from build123d import *

# Parameters (mm, degrees)
SKETCH1_W           = 97.5
SKETCH1_H           = 45.5
SKETCH1_W_2         = 93.5
SKETCH1_H_2         = 41.5
BOSS_EXTRUDE1_DEPTH = 4
SKETCH2_W           = 102.5
SKETCH2_H           = 50.5
BOSS_EXTRUDE2_DEPTH = 4
CUT_EXTRUDE1_DEPTH  = 58.689903796


with BuildPart() as part:
    # Sketch1 → Boss-Extrude1 (new body)
    with BuildSketch(Plane(origin=(0, 0, 0), x_dir=(1, 0, 0), z_dir=(0, 1, 0))):
        Rectangle(SKETCH1_W, SKETCH1_H)
        Rectangle(SKETCH1_W_2, SKETCH1_H_2, mode=Mode.SUBTRACT)
    extrude(amount=BOSS_EXTRUDE1_DEPTH)

    # Sketch2 → Boss-Extrude2 (add)
    with BuildSketch(Plane(origin=(0, 0, 0), x_dir=(-1, 0, 0), z_dir=(0, -1, 0))):
        Rectangle(SKETCH2_W, SKETCH2_H)
    extrude(amount=BOSS_EXTRUDE2_DEPTH)

    # Sketch3 → Cut-Extrude1 (cut, through all)
    with BuildSketch(Plane.XZ.offset(4)):
        with BuildLine():
            Line((21.754778505, -2.585841929), (14.396321324, 4.772615252))
            ThreePointArc((14.396321324, 4.772615252), (3.257355265, -2.585841929), (14.396321324, -9.94429911))
            Line((14.396321324, -9.94429911), (21.754778505, -2.585841929))
        make_face()
        with BuildLine():
            ThreePointArc((27.699814048, 16.344452811), (17.739587878, 15.654593104), (16.208809841, 5.78855386))
            Line((16.208809841, 5.78855386), (23.168992067, -1.171628366))
            Line((23.168992067, -1.171628366), (30.046481727, 5.705861294))
            ThreePointArc((30.046481727, 5.705861294), (31.14634131, 10.054344559), (29.732993239, 14.31127362))
            Line((29.732993239, 14.31127362), (27.699814048, 16.344452811))
        make_face()
        with BuildLine():
            ThreePointArc((15.482875978, -11.68617158), (23.435669898, -22.607420615), (29.929242502, -10.760305926))
            Line((29.929242502, -10.760305926), (23.168992067, -4.000055491))
            Line((23.168992067, -4.000055491), (15.482875978, -11.68617158))
        make_face()
        with BuildLine():
            ThreePointArc((40.538950668, 3.505316191), (36.33465085, 5.37848968), (31.79403897, 4.624991411))
            Line((31.79403897, 4.624991411), (24.58320563, -2.585841929))
            Line((24.58320563, -2.585841929), (31.677379035, -9.680015334))
            ThreePointArc((31.677379035, -9.680015334), (41.608009289, -7.500810005), (41.380693911, 2.663572949))
            Line((41.380693911, 2.663572949), (40.538950668, 3.505316191))
        make_face()
        with BuildLine():
            Line((-31.75, 0.342207976), (-38.75, 0.422889955))
            ThreePointArc((-38.75, 0.422889955), (-46.75, -7.577110045), (-38.75, -15.577110045))
            Line((-38.75, -15.577110045), (-8.75, -15.75))
            ThreePointArc((-8.75, -15.75), (-0.75, -7.75), (-8.75, 0.25))
            Line((-8.75, 0.25), (-15.75, 0.25))
            Line((-15.75, 0.25), (-15.75, 7.75))
            ThreePointArc((-15.75, 7.75), (-23.75, 15.75), (-31.75, 7.75))
            Line((-31.75, 7.75), (-31.75, 0.342207976))
        make_face()
    extrude(amount=-CUT_EXTRUDE1_DEPTH, mode=Mode.SUBTRACT)


solid = part.part
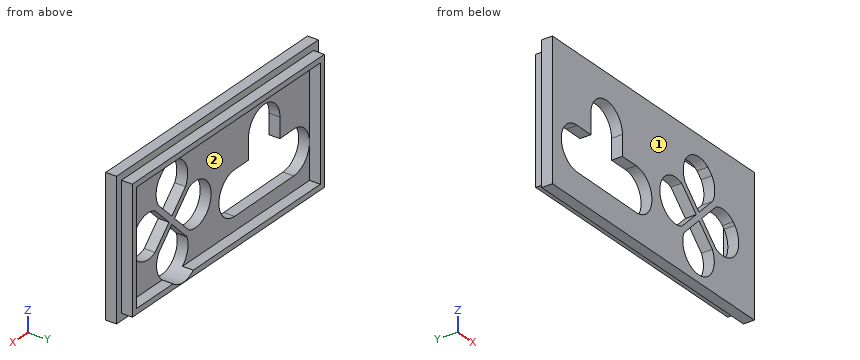
Build history of the part. All positions in model axes, mm. Face numbers are marked on the shaded views. Give positions to 0.01 mm unless a question says otherwise; leave off trailing zeros. Order: outer loops, then holes, each group sorted by start corner. A loop starts at its lowest first (then second) coordinate and runs counter-clockwise, first axis right, second up. Notation, with made-up numbers: M 83.25,68.25 L 116.25,68.25 A14 ccw 116.25,87.25 Z; hole C -39.5,-25.5 d2. An arc over 180 degrees is marked long. Put each result on its own line as item: value.
Item 1: Cut at D-D on x = -33. Write the cut outline in (y, z), then the cut area to 3 significant figures.
Results are:
outline: M -4,-25.25 L 0,-25.25 L 0,-22.75 L 4,-22.75 L 4,-20.75 L 0,-20.75 L 0,-15.61 L -4,-15.61 Z; M -4,0.36 L 0,0.36 L 0,20.75 L 4,20.75 L 4,22.75 L 0,22.75 L 0,25.25 L -4,25.25 Z
area: 154 mm2
Item 2: Cut at A-A on z = 10.5. Write the cut outline in (x, y).
Results are:
outline: M -51.25,-4 L -31.26,-4 L -31.26,0 L -46.75,0 L -46.75,4 L -48.75,4 L -48.75,0 L -51.25,0 Z; M -16.24,-4 L 15.19,-4 L 15.19,0 L -16.24,0 Z; M 31.12,-4 L 51.25,-4 L 51.25,0 L 48.75,0 L 48.75,4 L 46.75,4 L 46.75,0 L 31.12,0 Z
Item 3: Cut at B-B on y = -2.75. Write the cut outline in (x, z) (3 decimals), then the cut area to 3 significant figures.
Results are:
outline: M -51.25,-25.25 L 51.25,-25.25 L 51.25,25.25 L -51.25,25.25 Z; hole M -38.75,-15.577 L -8.75,-15.75 A8 ccw -8.75,0.25 L -15.75,0.25 L -15.75,7.75 A8 ccw -31.75,7.75 L -31.75,0.342 L -38.75,0.423 A8 ccw Z; hole M 14.396,-9.944 L 21.755,-2.586 L 14.396,4.773 A8 ccw long Z; hole M 15.483,-11.686 A8 ccw long 29.929,-10.76 L 23.169,-4 Z; hole M 16.209,5.789 L 23.169,-1.172 L 30.046,5.706 A8 ccw 29.733,14.311 L 27.7,16.344 A8 ccw Z; hole M 24.583,-2.586 L 31.677,-9.68 A8 ccw 41.381,2.664 L 40.539,3.505 A8 ccw 31.794,4.625 Z
area: 3,450 mm2
Item 4: Wall check: probe 1 along X at (y, z) = (1.25, 17.5); probe 2 along Z at (x, y) = (-8, 2); probe 3 along X at (y, z) = (-0.75, -6). Give the ranges that are in metal, low to high.
Results are:
probe 1: -48.75 to -46.75, 46.75 to 48.75
probe 2: -22.75 to -20.75, 20.75 to 22.75
probe 3: -51.25 to -46.59, -0.94 to 4.02, 18.34 to 21.17, 25.17 to 28, 42.54 to 51.25
Item 5: Pull direction Z, two halves, no side cores. Call the marked faces 1 and 2: +Z half, -Z half, draft (parallel to the pull), parting line (faces both ways), or undercut.
Results are:
face 1: draft
face 2: undercut
Item 6: Drop flat-ended pins along their axis: pin 1 Ø2 at (y, z) = (2, -20) entering from +X; pin 2 Ø4.5 at (x, y) = (-7, 2.5) entering from -Z; pin 3 Ø1.2 at (x, y) = (-25, 2) entering from +Z. Give the stop position or say it passes through.
Results are:
pin 1: x = 48.75
pin 2: z = -22.75
pin 3: z = 22.75
Item 7: Cut at C-C on x = 5. Write the cut outline in (y, z).
Results are:
outline: M -4,-25.25 L 0,-25.25 L 0,-22.75 L 4,-22.75 L 4,-20.75 L 0,-20.75 L 0,-7.57 L -4,-7.57 Z; M -4,2.4 L 0,2.4 L 0,20.75 L 4,20.75 L 4,22.75 L 0,22.75 L 0,25.25 L -4,25.25 Z
